Could you check a few things on this model? Use its own coordinates, in mm. A direction names the side the tool comes from. Round coordinates to 2 decimals unless told otherwise and drop trailing zeros. Loops run counter-clockwise (first coordinate to the right, second up) from the corner with the lowest first, then second, coordinate; pieces in that order, holes last. Notation, with made-up numbers: M 17,70.25 L 27,70.25 A33 ccw 27,104.25 Z; hole C 65,32 d2. An arc over 180 degrees is marked long. One line per item, written item: value. Start each with the question number.
Q1. Imagine slicing it at C-C (x = 325). Please give me the cut outline in (y, z), then the cut area to 3 significant figures.
Q2. Which directions (+Z, -Z, +X, -X, +Y, -Y) give clear straight access to the entire face, cutting with the end or side of a thin tool? Please do faces 1 (the face through (508, -1, 1)), 2 (the face through (254, 26.4, 58.2)), 3 (the face through (381, 26.4, 58.2)).
Q3. Imagine slicing it at D-D (y = 108). Please give me the cut outline in (x, z).
Q4. Imagine slicing it at A-A (y = 0). Please give me the cut outline in (x, z).
Q5. I'm going to push flat-ended pins straight in: pin 1 Ø8 at (x, z) = (380.5, 25.5) entering from -Y; pin 2 Ø10 at (x, z) = (378, 13.5) entering from -Y; pin 3 Ø1 at (x, z) = (147, -54.5) entering from -Y. Where does each tip first touch, or does it pass through?
Q6. Please list where these lines run through material, in increasing order: line 1 along X through (y, z) = (53, -97.5); line 2 along Z through (x, y) = (213, -2.5); line 3 along Z through (x, y) = (482.5, -38.5).
from build123d import *

# Parameters (mm, degrees)
F0_R     = 63.593416
F1_DEPTH = 508
F3_R     = 127
F4_DEPTH = 127


with BuildPart() as f1:
    # F0 (on Right) → F1 (new body)
    with BuildSketch(Plane.YZ):
        Circle(F0_R)
    extrude(amount=F1_DEPTH)

    # F3 (on offset) → F4 (join)
    with BuildSketch(Plane.YZ.offset(381)):
        Circle(F3_R)
    extrude(amount=-F4_DEPTH)


solid = f1.part
Report:
1. outline: C 0,0 d254
1. area: 50,700 mm²
2. face 1: +Z, -Z, +X, +Y, -Y
2. face 2: -X
2. face 3: +X
3. outline: M 254,-66.82 L 381,-66.82 L 381,66.82 L 254,66.82 Z
4. outline: M 0,-63.59 L 254,-63.59 L 254,-127 L 381,-127 L 381,-63.59 L 508,-63.59 L 508,63.59 L 381,63.59 L 381,127 L 254,127 L 254,63.59 L 0,63.59 Z
5. pin 1: stops at y = -125.17
5. pin 2: stops at y = -126.72
5. pin 3: stops at y = -33.59
6. line 1: x = 254 to 381
6. line 2: z = -63.54 to 63.54
6. line 3: z = -50.61 to 50.61
